Here's how the part is built. I have some questions about the finished solid (model axes, mm). A direction names the side the tool comes from. Coordinates: 2 decimals unless noted, no trailing zeros. Use a Markdown table: item, result.
```python
from build123d import *

# Parameters (mm, degrees)
F0_W     = 500
F0_H     = 30
F1_DEPTH = 300
F2_W     = 30
F2_H     = 30.000001
F3_DEPTH = 30
F4_W     = 30
F4_H     = 30
F5_DEPTH = 30


with BuildPart() as f1:
    # F0 (on Front) → F1 (new body)
    with BuildSketch(Plane.XZ):
        Rectangle(F0_W, F0_H)
    extrude(amount=F1_DEPTH)

    # F2 (on Front) → F3 (cut)
    with BuildSketch(Plane.XZ):
        with Locations((65, 0)):
            Rectangle(F2_W, F2_H)
    extrude(amount=F3_DEPTH, mode=Mode.SUBTRACT)

    # F4 (on Front) → F5 (cut)
    with BuildSketch(Plane.XZ):
        with Locations((-165, 0)):
            Rectangle(F4_W, F4_H)
    extrude(amount=F5_DEPTH, mode=Mode.SUBTRACT)


solid = f1.part
```
1. Which directions (+Z, -Z, +X, -X, +Y, -Y) give clear straight access to the entire face, cutting with the end or side of a thin tool? Please do faces 4 (the face through (-3, -148, -15)), 5 (the face through (50, -15, 0)).
Answers follow:
| item | result |
|---|---|
| face 4 | -Z, +X, -X, +Y, -Y |
| face 5 | +Z, -Z, +Y |
2. I need wall thicknesses on probe 1 along Y at (x, z) = (58, -4). Which ranges of the line are inside material? Lowest first, please.
Answers follow:
| item | result |
|---|---|
| probe 1 | y = -300 to -30 |
3. Will this pin go through, and if not, where does the flat tip stop? pin 1 Ø9 at (x, z) = (58, 1.5) entering from +Y.
Answers follow:
| item | result |
|---|---|
| pin 1 | stops at y = -30 |
4. We'd pull the mould along X, two halves only. Please class faces 1 (the face through (65, -30, 0)), 2 (the face through (250, -148, 0)), 3 (the face through (-3, -148, 15)): +X half, -X half, draft (parallel to the pull), parting line (faces both ways), or undercut.
Answers follow:
| item | result |
|---|---|
| face 1 | undercut |
| face 2 | +X half |
| face 3 | draft |
